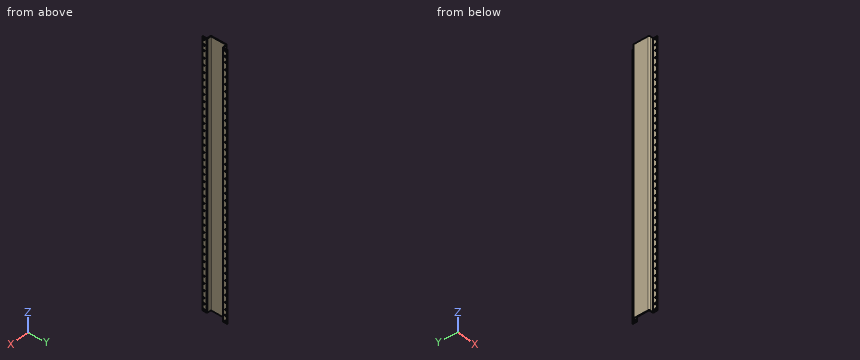
```python
from build123d import *

# Parameters (mm, degrees)
BRIDA_BASE5_DEPTH     = 1197.102
CROQUIS22_R           = 3.937
CORTAR_EXTRUIR1_DEPTH = 54.102
CROQUIS23_R           = 2.921
CORTAR_EXTRUIR2_DEPTH = 54.102


# Sheet-metal steps are written as plain solids
with BuildPart() as part:
    # Croquis1 → Brida base5 (new body)
    with BuildSketch(Plane.XY):
        with BuildLine():
            Line((0, 21.844), (0, 3.048))
            ThreePointArc((0, 3.048), (-0.892738531, 0.892738531), (-3.048, 0))
            Line((-3.048, 0), (-16.51, 0))
            ThreePointArc((-16.51, 0), (-18.665261469, -0.892738531), (-19.558, -3.048))
            Line((-19.558, -3.048), (-19.558, -67.564))
            ThreePointArc((-19.558, -67.564), (-18.665261469, -69.719261469), (-16.51, -70.612))
            Line((-16.51, -70.612), (-3.048, -70.612))
            ThreePointArc((-3.048, -70.612), (-0.892738531, -71.504738531), (0, -73.66))
            Line((0, -73.66), (0, -92.456))
            Line((0, -92.456), (-2.794, -92.456))
            Line((-2.794, -92.456), (-2.794, -73.66))
            ThreePointArc((-2.794, -73.66), (-2.868394878, -73.480394878), (-3.048, -73.406))
            Line((-3.048, -73.406), (-16.51, -73.406))
            ThreePointArc((-16.51, -73.406), (-20.640917816, -71.694917816), (-22.352, -67.564))
            Line((-22.352, -67.564), (-22.352, -3.048))
            ThreePointArc((-22.352, -3.048), (-20.640917816, 1.082917816), (-16.51, 2.794))
            Line((-16.51, 2.794), (-3.048, 2.794))
            ThreePointArc((-3.048, 2.794), (-2.868394878, 2.868394878), (-2.794, 3.048))
            Line((-2.794, 3.048), (-2.794, 21.844))
            Line((-2.794, 21.844), (0, 21.844))
        make_face()
    extrude(amount=BRIDA_BASE5_DEPTH)

    # Croquis22 → Cortar-Extruir1 (cut)
    with BuildSketch(Plane(origin=(0, 0, 0), x_dir=(0, 0, -1), z_dir=(1, 0, 0))):
        with Locations(Location((-1189.228, 13.891549634, 0), (0, 0, 90))):
            Circle(CROQUIS22_R)
        with Locations(Location((-1163.828, 13.891549634, 0), (0, 0, 90))):
            Circle(CROQUIS22_R)
        with Locations(Location((-1189.228, -84.582, 0), (0, 0, 90))):
            Circle(CROQUIS22_R)
        with Locations(Location((-1163.828, -84.582, 0), (0, 0, 90))):
            Circle(CROQUIS22_R)
        with Locations(Location((-7.874, 13.891549634, 0), (0, 0, 90))):
            Circle(CROQUIS22_R)
        with Locations(Location((-33.274, 13.891549634, 0), (0, 0, 90))):
            Circle(CROQUIS22_R)
        with Locations(Location((-7.874, -84.582, 0), (0, 0, 90))):
            Circle(CROQUIS22_R)
        with Locations(Location((-33.274, -84.582, 0), (0, 0, 90))):
            Circle(CROQUIS22_R)
    extrude(amount=-CORTAR_EXTRUIR1_DEPTH, mode=Mode.SUBTRACT)

    # Croquis23 → Cortar-Extruir2 (cut)
    with BuildSketch(Plane(origin=(0, 0, 0), x_dir=(0, 0, -1), z_dir=(1, 0, 0))):
        with Locations(Location((-1138.428, 13.891549634, 0), (0, 0, 90))):
            Circle(CROQUIS23_R)
        with Locations(Location((-1138.428, -84.582, 0), (0, 0, 90))):
            Circle(CROQUIS23_R)
        with Locations(Location((-1106.678, 13.891549634, 0), (0, 0, 90))):
            Circle(CROQUIS23_R)
        with Locations(Location((-1106.678, -84.582, 0), (0, 0, 90))):
            Circle(CROQUIS23_R)
        with Locations(Location((-1074.928, 13.891549634, 0), (0, 0, 90))):
            Circle(CROQUIS23_R)
        with Locations(Location((-1074.928, -84.582, 0), (0, 0, 90))):
            Circle(CROQUIS23_R)
        with Locations(Location((-1043.178, 13.891549634, 0), (0, 0, 90))):
            Circle(CROQUIS23_R)
        with Locations(Location((-1043.178, -84.582, 0), (0, 0, 90))):
            Circle(CROQUIS23_R)
        with Locations(Location((-1011.428, 13.891549634, 0), (0, 0, 90))):
            Circle(CROQUIS23_R)
        with Locations(Location((-1011.428, -84.582, 0), (0, 0, 90))):
            Circle(CROQUIS23_R)
        with Locations(Location((-979.678, 13.891549634, 0), (0, 0, 90))):
            Circle(CROQUIS23_R)
        with Locations(Location((-979.678, -84.582, 0), (0, 0, 90))):
            Circle(CROQUIS23_R)
        with Locations(Location((-947.928, 13.891549634, 0), (0, 0, 90))):
            Circle(CROQUIS23_R)
        with Locations(Location((-947.928, -84.582, 0), (0, 0, 90))):
            Circle(CROQUIS23_R)
        with Locations(Location((-916.178, 13.891549634, 0), (0, 0, 90))):
            Circle(CROQUIS23_R)
        with Locations(Location((-916.178, -84.582, 0), (0, 0, 90))):
            Circle(CROQUIS23_R)
        with Locations(Location((-884.428, 13.891549634, 0), (0, 0, 90))):
            Circle(CROQUIS23_R)
        with Locations(Location((-884.428, -84.582, 0), (0, 0, 90))):
            Circle(CROQUIS23_R)
        with Locations(Location((-852.678, 13.891549634, 0), (0, 0, 90))):
            Circle(CROQUIS23_R)
        with Locations(Location((-852.678, -84.582, 0), (0, 0, 90))):
            Circle(CROQUIS23_R)
        with Locations(Location((-820.928, 13.891549634, 0), (0, 0, 90))):
            Circle(CROQUIS23_R)
        with Locations(Location((-820.928, -84.582, 0), (0, 0, 90))):
            Circle(CROQUIS23_R)
        with Locations(Location((-789.178, 13.891549634, 0), (0, 0, 90))):
            Circle(CROQUIS23_R)
        with Locations(Location((-789.178, -84.582, 0), (0, 0, 90))):
            Circle(CROQUIS23_R)
        with Locations(Location((-757.428, 13.891549634, 0), (0, 0, 90))):
            Circle(CROQUIS23_R)
        with Locations(Location((-757.428, -84.582, 0), (0, 0, 90))):
            Circle(CROQUIS23_R)
        with Locations(Location((-725.678, 13.891549634, 0), (0, 0, 90))):
            Circle(CROQUIS23_R)
        with Locations(Location((-725.678, -84.582, 0), (0, 0, 90))):
            Circle(CROQUIS23_R)
        with Locations(Location((-693.928, 13.891549634, 0), (0, 0, 90))):
            Circle(CROQUIS23_R)
        with Locations(Location((-693.928, -84.582, 0), (0, 0, 90))):
            Circle(CROQUIS23_R)
        with Locations(Location((-662.178, 13.891549634, 0), (0, 0, 90))):
            Circle(CROQUIS23_R)
        with Locations(Location((-662.178, -84.582, 0), (0, 0, 90))):
            Circle(CROQUIS23_R)
        with Locations(Location((-630.428, 13.891549634, 0), (0, 0, 90))):
            Circle(CROQUIS23_R)
        with Locations(Location((-630.428, -84.582, 0), (0, 0, 90))):
            Circle(CROQUIS23_R)
        with Locations(Location((-598.678, 13.891549634, 0), (0, 0, 90))):
            Circle(CROQUIS23_R)
        with Locations(Location((-598.678, -84.582, 0), (0, 0, 90))):
            Circle(CROQUIS23_R)
        with Locations(Location((-566.928, 13.891549634, 0), (0, 0, 90))):
            Circle(CROQUIS23_R)
        with Locations(Location((-566.928, -84.582, 0), (0, 0, 90))):
            Circle(CROQUIS23_R)
        with Locations(Location((-535.178, 13.891549634, 0), (0, 0, 90))):
            Circle(CROQUIS23_R)
        with Locations(Location((-535.178, -84.582, 0), (0, 0, 90))):
            Circle(CROQUIS23_R)
        with Locations(Location((-503.428, 13.891549634, 0), (0, 0, 90))):
            Circle(CROQUIS23_R)
        with Locations(Location((-503.428, -84.582, 0), (0, 0, 90))):
            Circle(CROQUIS23_R)
        with Locations(Location((-471.678, 13.891549634, 0), (0, 0, 90))):
            Circle(CROQUIS23_R)
        with Locations(Location((-471.678, -84.582, 0), (0, 0, 90))):
            Circle(CROQUIS23_R)
        with Locations(Location((-439.928, 13.891549634, 0), (0, 0, 90))):
            Circle(CROQUIS23_R)
        with Locations(Location((-439.928, -84.582, 0), (0, 0, 90))):
            Circle(CROQUIS23_R)
        with Locations(Location((-408.178, 13.891549634, 0), (0, 0, 90))):
            Circle(CROQUIS23_R)
        with Locations(Location((-408.178, -84.582, 0), (0, 0, 90))):
            Circle(CROQUIS23_R)
        with Locations(Location((-376.428, 13.891549634, 0), (0, 0, 90))):
            Circle(CROQUIS23_R)
        with Locations(Location((-376.428, -84.582, 0), (0, 0, 90))):
            Circle(CROQUIS23_R)
        with Locations(Location((-344.678, 13.891549634, 0), (0, 0, 90))):
            Circle(CROQUIS23_R)
        with Locations(Location((-344.678, -84.582, 0), (0, 0, 90))):
            Circle(CROQUIS23_R)
        with Locations(Location((-312.928, 13.891549634, 0), (0, 0, 90))):
            Circle(CROQUIS23_R)
        with Locations(Location((-312.928, -84.582, 0), (0, 0, 90))):
            Circle(CROQUIS23_R)
        with Locations(Location((-281.178, 13.891549634, 0), (0, 0, 90))):
            Circle(CROQUIS23_R)
        with Locations(Location((-281.178, -84.582, 0), (0, 0, 90))):
            Circle(CROQUIS23_R)
        with Locations(Location((-249.428, 13.891549634, 0), (0, 0, 90))):
            Circle(CROQUIS23_R)
        with Locations(Location((-249.428, -84.582, 0), (0, 0, 90))):
            Circle(CROQUIS23_R)
        with Locations(Location((-217.678, 13.891549634, 0), (0, 0, 90))):
            Circle(CROQUIS23_R)
        with Locations(Location((-217.678, -84.582, 0), (0, 0, 90))):
            Circle(CROQUIS23_R)
        with Locations(Location((-185.928, 13.891549634, 0), (0, 0, 90))):
            Circle(CROQUIS23_R)
        with Locations(Location((-185.928, -84.582, 0), (0, 0, 90))):
            Circle(CROQUIS23_R)
        with Locations(Location((-154.178, 13.891549634, 0), (0, 0, 90))):
            Circle(CROQUIS23_R)
        with Locations(Location((-154.178, -84.582, 0), (0, 0, 90))):
            Circle(CROQUIS23_R)
        with Locations(Location((-122.428, 13.891549634, 0), (0, 0, 90))):
            Circle(CROQUIS23_R)
        with Locations(Location((-122.428, -84.582, 0), (0, 0, 90))):
            Circle(CROQUIS23_R)
        with Locations(Location((-90.678, 13.891549634, 0), (0, 0, 90))):
            Circle(CROQUIS23_R)
        with Locations(Location((-90.678, -84.582, 0), (0, 0, 90))):
            Circle(CROQUIS23_R)
        with Locations(Location((-58.928, 13.891549634, 0), (0, 0, 90))):
            Circle(CROQUIS23_R)
        with Locations(Location((-58.928, -84.582, 0), (0, 0, 90))):
            Circle(CROQUIS23_R)
    extrude(amount=-CORTAR_EXTRUIR2_DEPTH, mode=Mode.SUBTRACT)


solid = part.part
```
Source: CAD feature listing. Evaluate the final solid. Frame: model axes, mm. Coordinates: 2 decimals unless noted, no trailing zeros. Loops run counter-clockwise (first coordinate to the right, second up) from the corner with the lowest first, then second, coordinate; pieces in that order, holes last. Notation, with made-up numbers: (-22, 13.25) - (-5, 13.25) arc R10 cw to (-5, 29.25) - close; hole circle Ø4 at (-19, 14.25). An arc over 180 degrees is marked (long way). Answer as CSV lines item,"result".
1. Section B-B (y = -39.5). Return loops of the section in (x, z).
Established:
outline,"(-22.35, 0) - (-19.56, 0) - (-19.56, 1197.1) - (-22.35, 1197.1) - close"
2. Section A-A (x = -9.25). Return loops of the section in (y, z).
Established:
outline,"(-73.41, 0) - (-70.61, 0) - (-70.61, 1197.1) - (-73.41, 1197.1) - close; (0, 0) - (2.79, 0) - (2.79, 1197.1) - (0, 1197.1) - close"
3. Contact query for flat-ended pins moving along their axis: pin 1 (3.5 mm diameter, centred on y = -84.582, z = 1043.178, fed in from -X); pin 2 (5 mm diameter, centred on x = -5, z = 301, fed in from -Y); pin 3 (9.5 mm diameter, centred on y = 13.89, z = 439.93, fed in from -X); pin 4 (4 mm diameter, centred on y = -34, z = 405.5, fed in from +X). Output: stop coordinate, or through.
Established:
pin 1,"passes through"
pin 2,"stops at y = -92.46"
pin 3,"stops at x = -2.79"
pin 4,"stops at x = -19.56"
4. Ray query, line 1 (Y direction, x = -9.5, z = 666.5); line 2 (X direction, y = -21, z = 656); line 3 (X direction, y = 13, z = 1094.5). Return the intervals inside material, ascending.
Established:
line 1,"y = -73.41 to -70.61, 0 to 2.79"
line 2,"x = -22.35 to -19.56"
line 3,"x = -2.79 to 0"
